```python
from build123d import *

# Parameters (mm, degrees)
F0_W     = 5.000215
F0_H     = 10.000086
F1_DEPTH = 3


# Not quite as in the source:
# - ends of sketch curves that miss each other by under 0.0002 mm in the source are joined


with BuildPart() as f1:
    # F0 (on Right) → F1 (new body)
    with BuildSketch(Plane.YZ):
        Polygon((-27.499976, 19.999999), (-27.499976, -19.999998), (27.499976, -19.999998), (27.500024, 19.999999), (27.499976, 23.000002), (-27.499976, 23.000002), align=None)
        with Locations((22.1822251524, 1.1325399325)):
            Rectangle(F0_W, F0_H, mode=Mode.SUBTRACT)
    extrude(amount=F1_DEPTH)


solid = f1.part
```
Build history of the part. All positions in model axes, mm. A direction names the side the tool comes from. Round coordinates to 2 decimals unless told otherwise and drop trailing zeros. Order: outer loops, then holes, each group sorted by start corner. A loop starts at its lowest first (then second) coordinate and runs counter-clockwise, first axis right, second up. Notation, with made-up numbers: (-2.5, -29) -> (38.5, -29) arc R21 cw to (38.5, 4) -> close; hole circle Ø10 at (13.25, 35). An arc over 180 degrees is marked (long way). Answer in a Markdown table with one row per item.
1) Wall check: L1, parallel to Y at x = 0.5, z = 2.5. Give the ranges that are in metal, low to high.
Values:
| item | result |
|---|---|
| L1 | -27.5 to 19.68, 24.68 to 27.5 |
2) Band-saw the part on A-A on x = 1.45. Give the cut face in (y, z).
Values:
| item | result |
|---|---|
| outline | (-27.5, -20) -> (27.5, -20) -> (27.5, 20) -> (27.5, 23) -> (-27.5, 23) -> close; hole (19.68, -3.87) -> (24.68, -3.87) -> (24.68, 6.13) -> (19.68, 6.13) -> close |
3) Which spindle directions (+Z, -Z, +X, -X, +Y, -Y) get a long thin tool onto all of the face, cutting with end or side? Do faces 5 (the flat face through (3, 0, 2)), 6 (the flat face through (1, 22, 6.133)). Say none if no direction does.
Values:
| item | result |
|---|---|
| face 5 | +Z, -Z, +X, +Y, -Y |
| face 6 | +X, -X |
4) Mould opens along Z. For faces 1 (the flat face through (1, 22, -3.868)), 2 (the flat face through (1, 0, 23)), 3 (the flat face through (1, -27.5, 2)), 4 (the flat face through (1, 19.682, 1)) say: released by +Z, released by -Z, zero draft, split by the parting line, or undercut.
Values:
| item | result |
|---|---|
| face 1 | undercut |
| face 2 | released by +Z |
| face 3 | zero draft |
| face 4 | undercut |
